Geometry check sheet. Reference: the model listing, model coordinates, mm. A direction names the side the tool comes from. Give positions to 0.01 mm unless a question says otherwise; leave off trailing zeros. Order: outer loops, then holes, each group sorted by start corner. A loop starts at its lowest first (then second) coordinate and runs counter-clockwise, first axis right, second up. Notation, with made-up numbers: M -12,20 L 25,20 A18 ccw 25,48 Z; hole C -4,82.5 d10. An arc over 180 degrees is marked long. Answer as a JSON object with one key per item and string values. Group by question number.
from build123d import *

# Parameters (mm, degrees)
F0_W     = 73
F0_H     = 57
F1_DEPTH = 19
F2_T     = -2
F3_W     = 12.5
F3_H     = 11.5
F5_DEPTH = 25
F4_W     = 9.5
F4_H     = 11.5
F6_DEPTH = 25
F7_R     = 1


with BuildPart() as f1:
    # F0 (on Top) → F1 (new body)
    with BuildSketch(Plane.XY):
        Rectangle(F0_W, F0_H)
    extrude(amount=F1_DEPTH)

    # F2
    f2_openings = [f1.faces().sort_by_distance(p)[0] for p in [
        (0, 0, 19),
    ]]
    offset(amount=F2_T, openings=f2_openings)

    # F3 (on face) → F5 (cut)
    with BuildSketch(Plane.YZ.offset(36.5)):
        with Locations((-13.05, 10.75)):
            Rectangle(F3_W, F3_H)
    extrude(amount=-F5_DEPTH, mode=Mode.SUBTRACT)

    # F4 (on face) → F6 (cut)
    with BuildSketch(Plane.YZ.offset(36.5)):
        with Locations((19.75, 10.75)):
            Rectangle(F4_W, F4_H)
    extrude(amount=-F6_DEPTH, mode=Mode.SUBTRACT)

    # F7
    f7_edges = [f1.edges().sort_by_distance(p)[0] for p in [
        (0, -28.5, 0),
        (0, 28.5, 0),
        (-36.5, 0, 0),
        (36.5, -28.5, 9.5),
        (36.5, 0, 0),
        (-36.5, -28.5, 9.5),
        (36.5, 28.5, 9.5),
        (-36.5, 28.5, 9.5),
    ]]
    fillet(f7_edges, radius=F7_R)


solid = f1.part
1. Depth check by flat-ended pin: pin 1 (1.5 mm diameter, centred on x = 7, y = 10.5, fed in from +Z). Enter the tip coordinate at first touch or a pass-through.
2. Cross-section at C-C (x = -2.5). Record the cut outline in (y, z), and give its area (3 significant figures).
3. Release check for a two-part mould opening along Z. For faces 1 (the flat face through (0, -26.5, 10)), 2 (the flat face through (0, 0, 2)), 3 (the flat face through (36, 15, 11)) record: released by +Z, released by -Z, zero draft, split by the parting line, or undercut.
4. Cross-section at A-A (z = 13.5). Record the cut outline in (x, y), and give its area (3 significant figures).
5. Cross-section at D-D (y = -20.5). Record the cut outline in (x, z), and give its area (3 significant figures).
6. Thickness scan on line 1 along Y through (x, z) = (16, 13.25); line 2 along X through (y, z) = (1, 11.25); line 3 along Z through (x, y) = (-17, -9.5). Record the ranges inside material, lowest first. Write a range as [from, to].
7. Cross-section at B-B (y = -12.5). Record the cut outline in (x, z).
8. Access from +Z, -Z, +X, -X, +Y, -Y to the whole of each face (thin tool, end or side, straight path). Record for faces 4 (the flat face through (36, -6.8, 11)), 5 (the flat face through (0, 26.5, 10)), 6 (the flat face through (-3, -27, 19)).
Report:
{
 "1": {"pin 1": "stops at z = 2"},
 "2": {"outline": "M -28.5,1 A1 ccw -27.5,0 L 27.5,0 A1 ccw 28.5,1 L 28.5,19 L 26.5,19 L 26.5,2 L -26.5,2 L -26.5,19 L -28.5,19 Z", "area": "182 mm2"},
 "3": {"face 1": "zero draft", "face 2": "released by +Z", "face 3": "undercut"},
 "4": {"outline": "M -36.5,-27.5 A1 ccw -35.5,-28.5 L 35.5,-28.5 A1 ccw 36.5,-27.5 L 36.5,-19.3 L 34.5,-19.3 L 34.5,-26.5 L -34.5,-26.5 L -34.5,26.5 L 34.5,26.5 L 34.5,24.5 L 36.5,24.5 L 36.5,27.5 A1 ccw 35.5,28.5 L -35.5,28.5 A1 ccw -36.5,27.5 Z; M 34.5,-6.8 L 36.5,-6.8 L 36.5,15 L 34.5,15 Z", "area": "459 mm2"},
 "5": {"outline": "M -36.5,1 A1 ccw -35.5,0 L 35.5,0 A1 ccw 36.5,1 L 36.5,19 L 34.5,19 L 34.5,2 L -34.5,2 L -34.5,19 L -36.5,19 Z", "area": "214 mm2"},
 "6": {"line 1": "y = [-28.5, -26.5], [26.5, 28.5]", "line 2": "x = [-36.5, -34.5], [34.5, 36.5]", "line 3": "z = [0, 2]"},
 "7": {"outline": "M -36.5,1 A1 ccw -35.5,0 L 35.5,0 A1 ccw 36.5,1 L 36.5,5 L 34.5,5 L 34.5,2 L -34.5,2 L -34.5,19 L -36.5,19 Z; M 34.5,16.5 L 36.5,16.5 L 36.5,19 L 34.5,19 Z"},
 "8": {"face 4": "+X", "face 5": "+Z", "face 6": "+Z, +X, -X, +Y, -Y"}
}
